Geometry: final body of the model. Coordinates: model frame, mm. A direction names the side the tool comes from. Round coordinates to 2 decimals unless told otherwise and drop trailing zeros. Order: outer loops, then holes, each group sorted by start corner. A loop starts at its lowest first (then second) coordinate and runs counter-clockwise, first axis right, second up. Notation, with made-up numbers: (73.25, -26.75) -> (88.25, -26.75) arc R10 cw to (88.25, -16.75) -> close; hole circle Ø9 at (-17, 36). An arc over 180 degrees is marked (long way). Put each result on its own line as item: value.
```python
from build123d import *

# Parameters (mm, degrees)
SKIZZE1_R                            = 3.5
AUFSATZ_LINEAR_AUSTRAGEN1_DEPTH      = 90
SKIZZE3_R                            = 1.4
AUFSATZ_LINEAR_AUSTRAGEN2_DEPTH      = 4.9
AUFSATZ_LINEAR_START                 = 4.9
SKIZZE4_R                            = 1.4
AUFSATZ_LINEAR_AUSTRAGEN3_DEPTH      = 4.9
SCHNITT_LINEAR_AUSTRAGEN1_DEPTH      = 96.028995575
SCHNITT_LINEAR_AUSTRAGEN1_DEPTH_BACK = 96.028995575
SKIZZE5_W                            = 2
SKIZZE5_H                            = 8.003816725
SCHNITT_LINEAR_AUSTRAGEN2_DEPTH      = 96.023733877
SCHNITT_LINEAR_AUSTRAGEN2_DEPTH_BACK = 96.023733877
SKIZZE6_W                            = 3.926264937
SKIZZE6_H                            = 7.51599288


with BuildPart() as part:
    # Skizze1 → Aufsatz-Linear austragen1 (new body)
    with BuildSketch(Plane.XY):
        with Locations(Location((0, 0, 0), (0, 0, 180))):
            Circle(SKIZZE1_R)
    extrude(amount=AUFSATZ_LINEAR_AUSTRAGEN1_DEPTH)

    # Skizze3 → Aufsatz-Linear austragen2 (add)
    with BuildSketch(Plane.XY.offset(90)):
        Circle(SKIZZE3_R)
    extrude(amount=AUFSATZ_LINEAR_AUSTRAGEN2_DEPTH)

    # Skizze4 → Aufsatz-Linear austragen3 (add)
    with BuildSketch(Plane(origin=(0, 0, 0), x_dir=(-1, 0, 0), z_dir=(0, 0, -1)).offset(AUFSATZ_LINEAR_START)):
        with Locations(Location((0, 0, 0), (0, 0, 180))):
            Circle(SKIZZE4_R)
    extrude(amount=-AUFSATZ_LINEAR_AUSTRAGEN3_DEPTH)

    # Skizze5 → Schnitt-Linear austragen1 (cut, two sides: drawn at the far end of the back side and taken through both)
    with BuildSketch(Plane.XY.offset(90).offset(-SCHNITT_LINEAR_AUSTRAGEN1_DEPTH_BACK)):
        with Locations((0, -0.133552217)):
            Rectangle(SKIZZE5_W, SKIZZE5_H)
    extrude(amount=SCHNITT_LINEAR_AUSTRAGEN1_DEPTH + SCHNITT_LINEAR_AUSTRAGEN1_DEPTH_BACK, mode=Mode.SUBTRACT)


with BuildPart() as schnitt_linear_austragen1_piece_1:
    # of the separate pieces the step leaves, piece 1, a body of its own (schnitt_linear_austragen1_pieces)
    add(part.part.solids().sort_by_distance((-1, 3.354101966, 0))[0])


with BuildPart() as schnitt_linear_austragen1_piece_2:
    # of the separate pieces the step leaves, piece 2, a body of its own (schnitt_linear_austragen1_pieces)
    add(part.part.solids().sort_by_distance((1, -3.354101966, 0))[0])

    # Skizze6 → Schnitt-Linear austragen2 (cut, two sides: drawn at the far end of the back side and taken through both)
    with BuildSketch(Plane.XY.offset(90).offset(-SCHNITT_LINEAR_AUSTRAGEN2_DEPTH_BACK)):
        with Locations((2.16722224, 0.040063928)):
            Rectangle(SKIZZE6_W, SKIZZE6_H)
    extrude(amount=SCHNITT_LINEAR_AUSTRAGEN2_DEPTH + SCHNITT_LINEAR_AUSTRAGEN2_DEPTH_BACK, mode=Mode.SUBTRACT)


solid = schnitt_linear_austragen1_piece_1.part
```
1. Cut plane A-A on y = 0. Return loops of the section in (x, z), and give its area (3 significant figures).
Ans:
outline: (-3.5, 0) -> (-1.4, 0) -> (-1.4, -4.9) -> (-1, -4.9) -> (-1, 94.9) -> (-1.4, 94.9) -> (-1.4, 90) -> (-3.5, 90) -> close
area: 229 mm²
2. Contact query for flat-ended pins moving along their axis: P1, Ø1, axis at x = -3, y = 2, coming from the +Z side; P2, Ø1, axis at x = -2.5, z = 23.5, coming from the -Y side. Output: stop coordinate, or through.
Ans:
P1: z = 90
P2: y = -2.87
3. Cut plane C-C on z = 70. Return loops of the section in (x, y), and give its area (3 significant figures).
Ans:
outline: (-1, -3.35) -> (-1, 3.35) arc R3.5 ccw to start
area: 12.3 mm²
4. Cut plane B-B on x = -2.1. Return loops of the section in (y, z).
Ans:
outline: (-2.8, 0) -> (2.8, 0) -> (2.8, 90) -> (-2.8, 90) -> close
5. Set-up query: faces 1 (the face through (-1.4, 0, 92.4)), 2 (the face through (-1.4, 0, -2.5)), 3 (the face through (-3.5, 0.1, 44.4)). Return all of +Z, -Z, +X, -X, +Y, -Y with unobstructed straight access to the full face (end or side cutting, diameter ignored); none if empty.
Ans:
face 1: +Z, -X
face 2: -Z, -X
face 3: +Z, -Z, -X
6. Material intervals for probe 1 along Z at (x, y) = (-2.7, 1.5); probe 2 along X at (y, z) = (1, 6); probe 3 along X at (y, z) = (2.25, 15), sorted ascending.
Ans:
probe 1: 0 to 90
probe 2: -3.35 to -1
probe 3: -2.68 to -1
